```python
from build123d import *

# Parameters (mm, degrees)
F0_W     = 90.9334234893
F0_H     = 50.9791802615
F1_DEPTH = 300
F2_DEPTH = 600
F3_DEPTH = 200
F4_T     = -5


with BuildPart() as f1:
    # F0 (on Front) → F1 (new body)
    with BuildSketch(Plane.XZ):
        with Locations((2.5382172316, -42.5791377202)):
            Rectangle(F0_W, F0_H)
    extrude(amount=F1_DEPTH)

    # F2 (add): a face of the model
    f2_faces = [f1.faces().sort_by_distance(p)[0] for p in [
        (-42.928494513, -150, -42.5791377202),
    ]]
    extrude(f2_faces, amount=F2_DEPTH)

    # F3 (add): a face of the model
    f3_faces = [f1.faces().sort_by_distance(p)[0] for p in [
        (-297.4617827684, -150, -17.0895475894),
    ]]
    extrude(f3_faces, amount=F3_DEPTH)

    # F4
    f4_openings = [f1.faces().sort_by_distance(p)[0] for p in [
        (-297.461783, -150, 182.910452),
    ]]
    offset(amount=F4_T, openings=f4_openings)


solid = f1.part
```
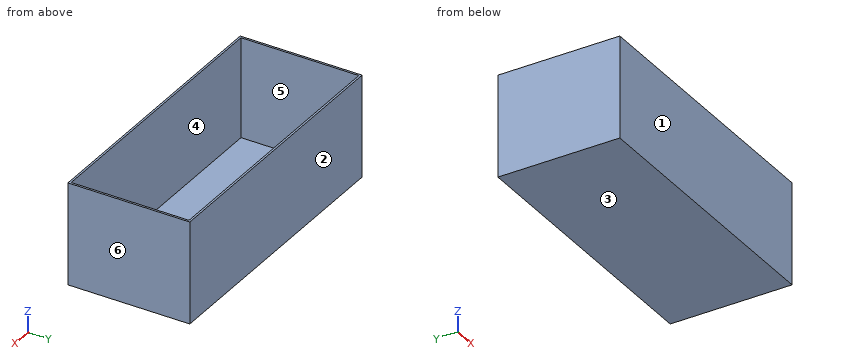
CAD build for the part. Positions are in the model's coordinates, mm. Face numbers are marked on the shaded views. A direction names the side the tool comes from. Round coordinates to 2 decimals unless told otherwise and drop trailing zeros. Loops run counter-clockwise (first coordinate to the right, second up) from the corner with the lowest first, then second, coordinate; pieces in that order, holes last. Notation, with made-up numbers: M -22,86.5 L 3,86.5 A9 cw 3,100.5 Z; hole C 85.25,3 d11. An arc over 180 degrees is marked long. Return JSON: item names as keys, results as strings. Group by question number.
(1) Wall check: probe 1 along Y at (x, z) = (-449, 143.5); probe 2 along X at (y, z) = (-153, 90); probe 3 along Z at (x, y) = (-449, -273.5). Give the ranges that are in metal, low to high. Write a range as [from, to].
(2) Drop a flat-ended pin along its axis: P1, Ø12, axis at x = -83, y = -165, coming from the +Z side. Give the stop position or say it passes through.
(3) Saw through at C-C, the plane x = -81. List the corners of the cut face in (y, z), and give its area (3 significant figures).
(4) Saw through at A-A, the plane z = 97.5. List the corners of the cut face in (x, y).
(5) Mould opens along Y. For the marked faces 1, 2, 3 and 4 say: +Y half, -Y half, draft (parallel to the pull), parting line (faces both ways), or undercut.
(6) Saw through at B-B, the plane y = -26. List the corners of the cut face in (x, z), and give its area (3 significant figures).
(7) Tool access for the marked faces 5 and 6: list every direction of +Z, -Z, +X, -X, +Y, -Y with a clear straight run to the whole face (end or side of a thin tool).
Answer list:
{
 "1": {"probe 1": "[-300, -295], [-5, 0]", "probe 2": "[-642.93, -637.93], [43, 48]", "probe 3": "[-68.07, -63.07]"},
 "2": {"P1": "z = -63.07"},
 "3": {"outline": "M -300,-68.07 L 0,-68.07 L 0,182.91 L -5,182.91 L -5,-63.07 L -295,-63.07 L -295,182.91 L -300,182.91 Z", "area": "3,960 mm2"},
 "4": {"outline": "M -642.93,-300 L 48,-300 L 48,0 L -642.93,0 Z; hole M -637.93,-295 L 43,-295 L 43,-5 L -637.93,-5 Z"},
 "5": {"face 1": "-Y half", "face 2": "+Y half", "face 3": "draft", "face 4": "undercut"},
 "6": {"outline": "M -642.93,-68.07 L 48,-68.07 L 48,182.91 L 43,182.91 L 43,-63.07 L -637.93,-63.07 L -637.93,182.91 L -642.93,182.91 Z", "area": "5,910 mm2"},
 "7": {"face 5": "+Z", "face 6": "+Z, -Z, +X, +Y, -Y"}
}
